from build123d import *

# Parameters (mm, degrees)
F1_DEPTH = 127
F3_DEPTH = 25.4
F4_R     = 3.81
F5_DEPTH = 25.4


with BuildPart() as f1:
    # F0 (on Front) → F1 (new body)
    with BuildSketch(Plane.XZ):
        with BuildLine():
            Line((-19.05, 44.45), (-19.05, 16.800521))
            ThreePointArc((-19.05, 16.800521), (-25.4, 0), (-19.05, -16.800521))
            Line((-19.05, -16.800521), (-19.05, -44.45))
            Line((-19.05, -44.45), (0, -44.45))
            Line((0, -44.45), (0, -17.7165))
            ThreePointArc((0, -17.7165), (-17.7165, 0), (0, 17.7165))
            Line((0, 17.7165), (0, 44.45))
            Line((0, 44.45), (-19.05, 44.45))
        make_face()
    extrude(amount=F1_DEPTH)

    # F2 (on face) → F3 (cut)
    with BuildSketch(Plane(origin=(-19.05, 0, 0), x_dir=(0, -1, 0), z_dir=(-1, 0, 0))):
        with BuildLine():
            ThreePointArc((67.31, -30.62526), (66.194077, -27.931184), (63.5, -26.81526))
            Line((63.5, -26.81526), (63.5, -34.43526))
            ThreePointArc((63.5, -34.43526), (66.194077, -33.319337), (67.31, -30.62526))
        make_face()
        with BuildLine():
            Line((63.5, -34.43526), (63.5, -26.81526))
            ThreePointArc((63.5, -26.81526), (59.69, -30.62526), (63.5, -34.43526))
        make_face()
        with BuildLine():
            ThreePointArc((35.56, -30.62526), (34.444077, -27.931184), (31.75, -26.81526))
            Line((31.75, -26.81526), (31.75, -34.43526))
            ThreePointArc((31.75, -34.43526), (34.444077, -33.319337), (35.56, -30.62526))
        make_face()
        with BuildLine():
            Line((31.75, -34.43526), (31.75, -26.81526))
            ThreePointArc((31.75, -26.81526), (27.94, -30.62526), (31.75, -34.43526))
        make_face()
        with BuildLine():
            ThreePointArc((95.25, -34.43526), (97.944077, -33.319337), (99.06, -30.62526))
            ThreePointArc((99.06, -30.62526), (97.944077, -27.931184), (95.25, -26.81526))
            Line((95.25, -26.81526), (95.25, -34.43526))
        make_face()
        with BuildLine():
            Line((95.25, -34.43526), (95.25, -26.81526))
            ThreePointArc((95.25, -26.81526), (91.44, -30.62526), (95.25, -34.43526))
        make_face()
    extrude(amount=-F3_DEPTH, mode=Mode.SUBTRACT)

    # F4 (on face) → F5 (cut)
    with BuildSketch(Plane(origin=(-19.05, 0, 0), x_dir=(0, -1, 0), z_dir=(-1, 0, 0))):
        with BuildLine():
            ThreePointArc((63.5, 26.81526), (66.194077, 27.931184), (67.31, 30.62526))
            ThreePointArc((67.31, 30.62526), (66.194077, 33.319337), (63.5, 34.43526))
            Line((63.5, 34.43526), (63.5, 26.81526))
        make_face()
        with BuildLine():
            Line((63.5, 26.81526), (63.5, 34.43526))
            ThreePointArc((63.5, 34.43526), (59.69, 30.62526), (63.5, 26.81526))
        make_face()
        with Locations((31.75, 30.62526)):
            Circle(F4_R)
        with Locations((95.25, 30.62526)):
            Circle(F4_R)
    extrude(amount=-F5_DEPTH, mode=Mode.SUBTRACT)


solid = f1.part
Model file for the job. Use its own axes, mm. A direction names the side the tool comes from. Give positions to 0.01 mm unless a question says otherwise; leave off trailing zeros. Order: outer loops, then holes, each group sorted by start corner. A loop starts at its lowest first (then second) coordinate and runs counter-clockwise, first axis right, second up. Notation, with made-up numbers: (-29, 34) - (13, 34) arc R27 ccw to (13, 54) - close; hole circle Ø3 at (60, 50.25). An arc over 180 degrees is marked (long way). Return JSON: item names as keys, results as strings.
1) Pull direction Z, two halves, no side cores. Call faces 4 (the flat face through (-19, -127, 1)), 5 (the cylindrical face through (-17.712, -62.611, -0.39)), 6 (the flat face through (-10, -63, -44.45)): pulls with the +Z half, pulls with the -Z half, needs draft (parallel to the pull), parting line crosses it, or undercut.
Geometry says:
{"face 4": "needs draft", "face 5": "undercut", "face 6": "pulls with the -Z half"}
2) Flat gauge pins, fed straight in: P1, Ø22, axis at y = -64.5, z = -29.5, coming from the -X side; P2, Ø6, axis at y = -31.75, z = 30.63, coming from the -X side; P3, Ø5, axis at y = -94.5, z = -1, coming from the -X side. Where does each tip first touch, or does it go through?
Geometry says:
{"P1": "x = -19.05", "P2": "through", "P3": "x = -25.4"}
3) Cut at D-D, the plane z = 0. Give the cut face in (x, y).
Geometry says:
{"outline": "(-25.4, -127) - (-17.72, -127) - (-17.72, 0) - (-25.4, 0) - close"}
4) Cut at A-A, the plane x = -7.75. Give the cut face in (y, z).
Geometry says:
{"outline": "(-127, -44.45) - (0, -44.45) - (0, -15.93) - (-127, -15.93) - close; (-127, 15.93) - (0, 15.93) - (0, 44.45) - (-127, 44.45) - close; hole (-99.06, -30.63) arc R3.81 ccw (long way) to (-95.25, -26.82) arc R3.81 ccw to start; hole circle Ø7.62 at (-95.25, 30.63); hole (-67.31, -30.63) arc R3.81 ccw (long way) to (-63.5, -26.82) arc R3.81 ccw to start; hole (-67.31, 30.63) arc R3.81 ccw to (-63.5, 26.82) arc R3.81 ccw (long way) to start; hole (-35.56, -30.63) arc R3.81 ccw (long way) to (-31.75, -26.82) arc R3.81 ccw to start; hole circle Ø7.62 at (-31.75, 30.63)"}
5) Cut at C-C, the plane z = 29. Give the cut face in (x, y).
Geometry says:
{"outline": "(-19.05, -127) - (0, -127) - (0, -98.7) - (-19.05, -98.7) - close; (-19.05, -91.8) - (0, -91.8) - (0, -66.95) - (-19.05, -66.95) - close; (-19.05, -60.05) - (0, -60.05) - (0, -35.2) - (-19.05, -35.2) - close; (-19.05, -28.3) - (0, -28.3) - (0, 0) - (-19.05, 0) - close"}
6) Probe line 1 (Z direction, x = -11, y = -95.25); line 2 (Z direction, x = -9, y = -96); line 3 (X direction, y = -53.5, z = -32). List the from-to ranges inside material, lowest first. Write a range as from..to.
Geometry says:
{"line 1": "-44.45..-34.44, -26.82..-13.89, 13.89..26.82, 34.44..44.45", "line 2": "-44.45..-34.36, -26.89..-15.26, 15.26..26.89, 34.36..44.45", "line 3": "-19.05..0"}
7) 3-axis set-ups, long thin cutter, end or side, ignore diameter. For faces 1 (the flat face through (-19.05, -63, 37)), 2 (the flat face through (-19.05, -63, -24)), 3 (the cylindrical face through (-9.658, -33.508, 27.245)): which of +Z, -Z, +X, -X, +Y, -Y reach the whole face in a straight line?
Geometry says:
{"face 1": "+Z, -X, +Y, -Y", "face 2": "-Z, -X, +Y, -Y", "face 3": "+X, -X"}
8) Cut at B-B, the plane y = -76. Give the cut face in (x, z).
Geometry says:
{"outline": "(-19.05, -44.45) - (0, -44.45) - (0, -17.72) arc R17.72 cw to (0, 17.72) - (0, 44.45) - (-19.05, 44.45) - (-19.05, 16.8) arc R25.4 ccw to (-19.05, -16.8) - close"}
